Could you check a few things on this drawing? It's one solid part, dimensions in mm from its lowest x, y, z. A direction names the side the tool comes from. Coordinates: 2 decimals unless noted, no trailing zeros. Order: outer loops, then holes, each group sorted by start corner. A loop starts at its lowest first (then second) coordinate and runs counter-clockwise, first axis right, second up. Notation, with made-up numbers: (48.5, 33) - (83.5, 33) arc R18 ccw to (83.5, 46) - close; hole circle Ø10 at (-31.5, 68). An arc over 180 degrees is marked (long way). Answer in a Markdown table with one row per item. Add a question column.
Item 1: I want a section at B-B (z = 1.3). Please give me the cut outline in (x, y), plus the area to 3 significant figures.
Item 2: Will these pins go through, and if not, where does the flat tip stop? pin 1 Ø0.6 at (y, z) = (1, 1.5) entering from -X; pin 2 Ø1.5 at (x, y) = (3.5, 1) entering from -Z.
Item 3: I want a section at C-C (x = 4.85). Please give me the cut outline in (y, z).
Item 4: If I drill on line 1 along Y through (x, z) = (4.1, 1.45) (1 decimal); line 2 along Z through (x, y) = (1.35, 3); line 3 along X through (y, z) = (1, 1.15), over which ranges is the centre line in solid material (lowest first)? Write a range as from..to.
Item 5: I want a section at D-D (x = 1.8). Please give me the cut outline in (y, z).
Item 6: Thinking about a two-plate mould opening in Y: for the marked faces 1, 2 and 3, which applies, +Y half, -Y half, draft (parallel to the pull), parting line (faces both ways), or undercut?
Item 7: I want a section at A-A (y = 1). Please give me the cut outline in (x, z), plus the area to 3 significant figures.
Item 8: On a 3-axis mill with a long thin cutter (end or side, diameter ignored), from which of +Z, -Z, +X, -X, +Y, -Y can I reach the whole of each face in a straight line? I mean the marked faces 4 and 5. Say none if no direction works.
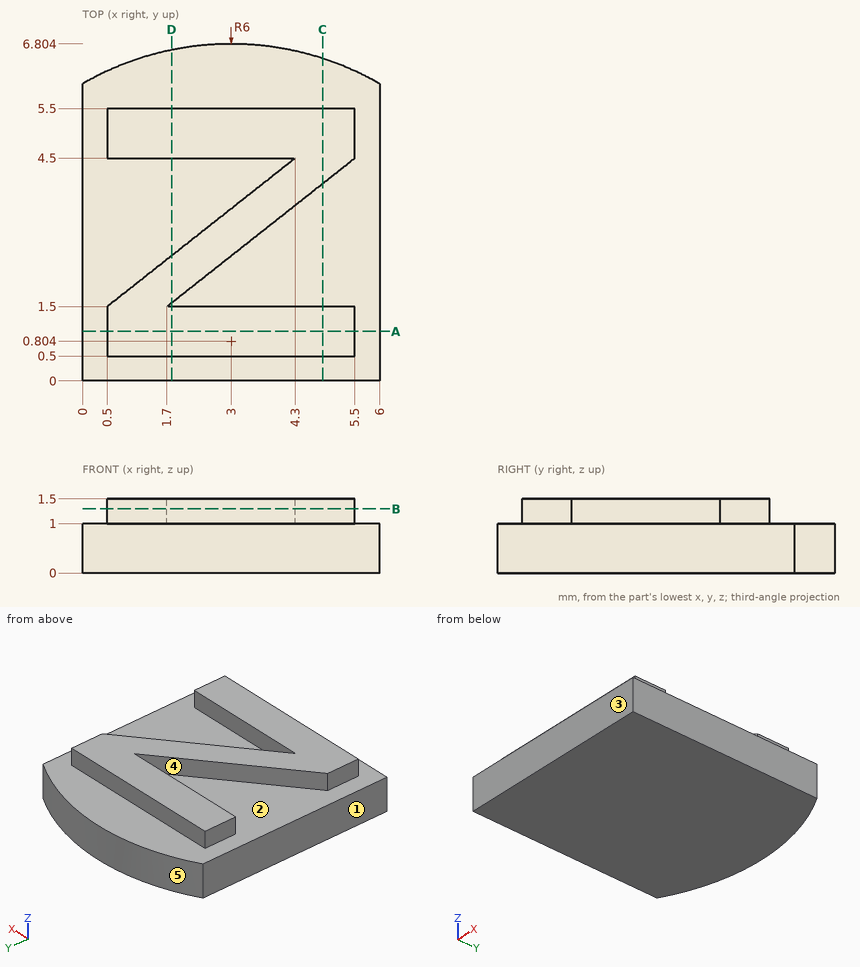
Values follow:
| question | item | result |
|---|---|---|
| 1 | outline | (0.5, 0.5) - (5.5, 0.5) - (5.5, 1.5) - (1.7, 1.5) - (5.5, 4.5) - (5.5, 5.5) - (0.5, 5.5) - (0.5, 4.5) - (4.3, 4.5) - (0.5, 1.5) - close |
| 1 | area | 13.6 mm^2 |
| 2 | pin 1 | stops at x = 0.5 |
| 2 | pin 2 | stops at z = 0 |
| 3 | outline | (0, 0) - (6.51, 0) - (6.51, 1) - (5.5, 1) - (5.5, 1.5) - (3.99, 1.5) - (3.99, 1) - (1.5, 1) - (1.5, 1.5) - (0.5, 1.5) - (0.5, 1) - (0, 1) - close |
| 4 | line 1 | y = 0.5..1.5, 3.4..4.3, 4.5..5.5 |
| 4 | line 2 | z = 0..1 |
| 4 | line 3 | x = 0.5..5.5 |
| 5 | outline | (0, 0) - (6.68, 0) - (6.68, 1) - (5.5, 1) - (5.5, 1.5) - (4.5, 1.5) - (4.5, 1) - (2.53, 1) - (2.53, 1.5) - (1.58, 1.5) - (1.58, 1) - (1.5, 1) - (1.5, 1.5) - (0.5, 1.5) - (0.5, 1) - (0, 1) - close |
| 6 | face 1 | draft |
| 6 | face 2 | undercut |
| 6 | face 3 | -Y half |
| 7 | outline | (0, 0) - (6, 0) - (6, 1) - (5.5, 1) - (5.5, 1.5) - (0.5, 1.5) - (0.5, 1) - (0, 1) - close |
| 7 | area | 8.50 mm^2 |
| 8 | face 4 | +Z, -X |
| 8 | face 5 | +Z, -Z, +Y |
